Read the model definition and answer for the solid it produces. Units are mm, in the model's axes. A direction names the side the tool comes from. Round coordinates to 2 decimals unless told otherwise and drop trailing zeros. Order: outer loops, then holes, each group sorted by start corner. A loop starts at its lowest first (then second) coordinate and runs counter-clockwise, first axis right, second up. Notation, with made-up numbers: (84, 42.25) -> (127, 42.25) arc R23 ccw to (127, 77.25) -> close; hole circle Ø3 at (26, 67.25). An arc over 180 degrees is marked (long way). Answer as a JSON object with one key per item and string values. Group by question number.
Item 1: Consider probe 1 along X at (y, z) = (-0.25, 3.25); probe 2 along Y at (x, z) = (-29, 3.25); probe 3 along X at (y, z) = (4.75, 7.25). Determine where each line is inside the solid, lowest interval first. Write a range as from..to.
Item 2: The mould has two halves that part along Y. Classify faces 1 (the cylindrical face through (-60.535, -0.806, 5.265)), 2 (the flat face through (63, 0, 6)), 3 (the flat face through (-1, -9.52, 5)): pulls with the +Y half, pulls with the -Y half, needs draft (parallel to the pull), parting line crosses it, or undercut.
Item 3: Section D-D, the plane y = -5.25 is taken. Write down the section's boundary in (x, z), plus the area to 3 significant figures.
Item 4: Section B-B, the plane z = 4 is taken. Write down the section's boundary in (x, y), plus the area to 3 significant figures.
Item 5: Given P1, Ø1.5, axis at y = 0, z = 3.5, coming from the +X side, flat-ended and moving along its own axis, determine where the tip first touches the part or whether it passes through.
Item 6: Section C-C, the plane y = 0 is taken. Write down the section's boundary in (x, z), plus the area to 3 significant figures.
Item 7: For faces 4 (the flat face through (-58, 0, 4)), 5 (the flat face through (-1, 9.52, 5)), 6 (the cylindrical face through (60.535, 0.806, 5.265)), determine the directions among +Z, -Z, +X, -X, +Y, -Y from which every point of the face is accessible in a straight line to the end or side of a thin tool.
Item 8: Section A-A, the plane x = 31 is taken. Write down the section's boundary in (y, z), plus the area to 3 significant figures.
from build123d import *

# Parameters (mm, degrees)
F0_W     = 126
F0_H     = 19.04
F1_DEPTH = 9.5
F2_R     = 1.5
F3_DEPTH = 5
F4_R     = 1.5
F5_DEPTH = 5
F6_R     = 8.02
F7_DEPTH = 9.5


with BuildPart() as f1:
    # F0 (on Top) → F1 (new body)
    with BuildSketch(Plane.XY):
        Rectangle(F0_W, F0_H)
    extrude(amount=F1_DEPTH)

    # F2 (on face) → F3 (cut)
    with BuildSketch(Plane(origin=(-63, 0, 0), x_dir=(0, -1, 0), z_dir=(-1, 0, 0))):
        with Locations((0, 4)):
            Circle(F2_R)
    extrude(amount=-F3_DEPTH, mode=Mode.SUBTRACT)

    # F4 (on face) → F5 (cut)
    with BuildSketch(Plane.YZ.offset(63)):
        with Locations((0, 4)):
            Circle(F4_R)
    extrude(amount=-F5_DEPTH, mode=Mode.SUBTRACT)

    # F6 (on face) → F7 (cut)
    with BuildSketch(Plane.XY.offset(9.5)):
        with Locations((-29, 0)):
            Circle(F6_R)
        with Locations((31, 0)):
            Circle(F6_R)
    extrude(amount=-F7_DEPTH, mode=Mode.SUBTRACT)


solid = f1.part
Values found:
{
 "1": {"probe 1": "-58..-37.02, -20.98..22.98, 39.02..58", "probe 2": "-9.52..-8.02, 8.02..9.52", "probe 3": "-63..-35.46, -22.54..24.54, 37.46..63"},
 "2": {"face 1": "undercut", "face 2": "needs draft", "face 3": "pulls with the -Y half"},
 "3": {"outline": "(-63, 0) -> (-35.06, 0) -> (-35.06, 9.5) -> (-63, 9.5) -> close; (-22.94, 0) -> (24.94, 0) -> (24.94, 9.5) -> (-22.94, 9.5) -> close; (37.06, 0) -> (63, 0) -> (63, 9.5) -> (37.06, 9.5) -> close", "area": "967 mm2"},
 "4": {"outline": "(-63, -9.52) -> (63, -9.52) -> (63, -1.5) -> (58, -1.5) -> (58, 1.5) -> (63, 1.5) -> (63, 9.52) -> (-63, 9.52) -> (-63, 1.5) -> (-58, 1.5) -> (-58, -1.5) -> (-63, -1.5) -> close; hole circle Ø16.04 at (-29, 0); hole circle Ø16.04 at (31, 0)", "area": "1,960 mm2"},
 "5": {"P1": "x = 58"},
 "6": {"outline": "(-63, 0) -> (-37.02, 0) -> (-37.02, 9.5) -> (-63, 9.5) -> (-63, 5.5) -> (-58, 5.5) -> (-58, 2.5) -> (-63, 2.5) -> close; (-20.98, 0) -> (22.98, 0) -> (22.98, 9.5) -> (-20.98, 9.5) -> close; (39.02, 0) -> (63, 0) -> (63, 2.5) -> (58, 2.5) -> (58, 5.5) -> (63, 5.5) -> (63, 9.5) -> (39.02, 9.5) -> close", "area": "862 mm2"},
 "7": {"face 4": "-X", "face 5": "+Z, -Z, +X, -X, +Y", "face 6": "+X"},
 "8": {"outline": "(-9.52, 0) -> (-8.02, 0) -> (-8.02, 9.5) -> (-9.52, 9.5) -> close; (8.02, 0) -> (9.52, 0) -> (9.52, 9.5) -> (8.02, 9.5) -> close", "area": "28.5 mm2"}
}
